Could you check a few things on this model? Use its own coordinates, in mm. A direction names the side the tool comes from. Give positions to 0.01 mm unless a question says otherwise; leave off trailing zeros. Loops run counter-clockwise (first coordinate to the right, second up) from the corner with the lowest first, then second, coordinate; pieces in that order, holes last. Notation, with made-up numbers: (-4.5, 66.25) - (19.5, 66.25) arc R29 ccw to (19.5, 104.25) - close; hole circle Ø3 at (-24, 39). An arc over 180 degrees is marked (long way). Answer in a Markdown table with one row per item. Add a question column.
```python
from build123d import *

# Parameters (mm, degrees)
F0_W          = 152
F0_H          = 55
F1_DEPTH      = 39
F2_W          = 53
F2_H          = 34
F3_DEPTH      = 150
F5_DEPTH      = 10.9
F7_DEPTH      = 100
F8_DEPTH      = 5
F9_DEPTH      = 4
F10_DEPTH     = 5
F11_DEPTH     = 5
F12_DEPTH     = 5
F13_W         = 8
F13_H         = 4
F14_DEPTH     = 100
F15_T1_DEPTH  = 163.5
F15_T3_DEPTH  = 74
F15_T5_DEPTH  = 56.5
F15_T7_DEPTH  = 55
F15_S11_W     = 5
F15_S11_H     = 5
F15_T12_DEPTH = 5
F15_S17_W     = 5
F15_S17_H     = 5
F15_T18_DEPTH = 5
F16_W         = 7.2434431314
F16_H         = 13.5
F16_W_2       = 55
F16_W_3       = 10.0454574823
F17_DEPTH     = 6
F18_R         = 5
F19_W         = 10
F19_H         = 4
F20_DEPTH     = 38.8


# Not quite as in the source:
# - a fillet or chamfer that OpenCascade refuses, or shapes differently, is made with other operations: its cross-section is extruded or revolved along the edge and cut away or added


with BuildPart() as f1:
    # F0 (on Top) → F1 (new body)
    with BuildSketch(Plane.XY):
        Rectangle(F0_W, F0_H)
    extrude(amount=F1_DEPTH)

    # F2 (on face) → F3 (cut)
    with BuildSketch(Plane(origin=(-76, 0, 0), x_dir=(0, -1, 0), z_dir=(-1, 0, 0))):
        with Locations((0, 19.5)):
            Rectangle(F2_W, F2_H)
    extrude(amount=-F3_DEPTH, mode=Mode.SUBTRACT)

    # F4 (on face) → F5 (cut)
    with BuildSketch(Plane(origin=(0, 0, 0), x_dir=(1, 0, 0), z_dir=(0, 0, -1))):
        with BuildLine():
            ThreePointArc((-29.5, 16.5), (-30.9644660941, 20.0355339059), (-34.5, 21.5))
            Line((-34.5, 21.5), (-59.5, 21.5))
            ThreePointArc((-59.5, 21.5), (-63.0355339059, 20.0355339059), (-64.5, 16.5))
            Line((-64.5, 16.5), (-64.5, -16.5))
            ThreePointArc((-64.5, -16.5), (-63.0355339059, -20.0355339059), (-59.5, -21.5))
            Line((-59.5, -21.5), (-34.5, -21.5))
            ThreePointArc((-34.5, -21.5), (-30.9644660941, -20.0355339059), (-29.5, -16.5))
            Line((-29.5, -16.5), (-29.5, 16.5))
        make_face()
        with BuildLine():
            Line((-12.5, -21.5), (12.5, -21.5))
            ThreePointArc((12.5, -21.5), (16.0355339059, -20.0355339059), (17.5, -16.5))
            Line((17.5, -16.5), (17.5, 16.5))
            ThreePointArc((17.5, 16.5), (16.0355339059, 20.0355339059), (12.5, 21.5))
            Line((12.5, 21.5), (-12.5, 21.5))
            ThreePointArc((-12.5, 21.5), (-16.0355339059, 20.0355339059), (-17.5, 16.5))
            Line((-17.5, 16.5), (-17.5, -16.5))
            ThreePointArc((-17.5, -16.5), (-16.0355339059, -20.0355339059), (-12.5, -21.5))
        make_face()
        with BuildLine():
            ThreePointArc((64.5, 16.5), (63.0355339059, 20.0355339059), (59.5, 21.5))
            Line((59.5, 21.5), (34.5, 21.5))
            ThreePointArc((34.5, 21.5), (30.9644660941, 20.0355339059), (29.5, 16.5))
            Line((29.5, 16.5), (29.5, -16.5))
            ThreePointArc((29.5, -16.5), (30.9644660941, -20.0355339059), (34.5, -21.5))
            Line((34.5, -21.5), (59.5, -21.5))
            ThreePointArc((59.5, -21.5), (63.0355339059, -20.0355339059), (64.5, -16.5))
            Line((64.5, -16.5), (64.5, 16.5))
        make_face()
    extrude(amount=-F5_DEPTH, mode=Mode.SUBTRACT)

    # F6 (on face) → F7 (cut)
    with BuildSketch(Plane.XZ.offset(27.5)):
        with BuildLine():
            ThreePointArc((-28, 29.5), (-29.4644660941, 33.0355339059), (-33, 34.5))
            Line((-33, 34.5), (-63, 34.5))
            ThreePointArc((-63, 34.5), (-66.5355339059, 33.0355339059), (-68, 29.5))
            Line((-68, 29.5), (-68, 9.5))
            ThreePointArc((-68, 9.5), (-66.5355339059, 5.9644660941), (-63, 4.5))
            Line((-63, 4.5), (-33, 4.5))
            ThreePointArc((-33, 4.5), (-29.4644660941, 5.9644660941), (-28, 9.5))
            Line((-28, 9.5), (-28, 29.5))
        make_face()
        with BuildLine():
            ThreePointArc((20, 29.5), (18.5355339059, 33.0355339059), (15, 34.5))
            Line((15, 34.5), (-15, 34.5))
            ThreePointArc((-15, 34.5), (-18.5355339059, 33.0355339059), (-20, 29.5))
            Line((-20, 29.5), (-20, 9.5))
            ThreePointArc((-20, 9.5), (-18.5355339059, 5.9644660941), (-15, 4.5))
            Line((-15, 4.5), (15, 4.5))
            ThreePointArc((15, 4.5), (18.5355339059, 5.9644660941), (20, 9.5))
            Line((20, 9.5), (20, 29.5))
        make_face()
        with BuildLine():
            ThreePointArc((58, 29.5), (56.5355339059, 33.0355339059), (53, 34.5))
            Line((53, 34.5), (33, 34.5))
            ThreePointArc((33, 34.5), (29.4644660941, 33.0355339059), (28, 29.5))
            Line((28, 29.5), (28, 9.5))
            ThreePointArc((28, 9.5), (29.4644660941, 5.9644660941), (33, 4.5))
            Line((33, 4.5), (53, 4.5))
            ThreePointArc((53, 4.5), (56.5355339059, 5.9644660941), (58, 9.5))
            Line((58, 9.5), (58, 29.5))
        make_face()
    extrude(amount=-F7_DEPTH, mode=Mode.SUBTRACT)

    # F8 (add): a face of the model
    f8_faces = [f1.faces().sort_by_distance(p)[0] for p in [
        (0, 0, 39),
    ]]
    extrude(f8_faces, amount=F8_DEPTH)

    # F9 (add): a face of the model
    f9_faces = [f1.faces().sort_by_distance(p)[0] for p in [
        (76, 0, 22),
    ]]
    extrude(f9_faces, amount=F9_DEPTH)

    # F10 (add): a face of the model
    f10_faces = [f1.faces().sort_by_distance(p)[0] for p in [
        (2, 0, 44),
    ]]
    extrude(f10_faces, amount=F10_DEPTH)

    # F11 (add): a face of the model
    f11_faces = [f1.faces().sort_by_distance(p)[0] for p in [
        (-74.3648547465, 27.5, 24.5),
    ]]
    extrude(f11_faces, amount=F11_DEPTH)

    # F12 (add): a face of the model
    f12_faces = [f1.faces().sort_by_distance(p)[0] for p in [
        (-74.3648547465, -27.5, 24.5),
    ]]
    extrude(f12_faces, amount=F12_DEPTH)

    # F13 (on face) → F14 (cut)
    with BuildSketch(Plane.XZ.offset(32.5)):
        with Locations((-26, 43.8039299548)):
            Rectangle(F13_W, F13_H)
        with Locations((10, 43.8039299548)):
            Rectangle(F13_W, F13_H)
        with Locations((63, 43.8039299548)):
            Rectangle(F13_W, F13_H)
    extrude(amount=-F14_DEPTH, mode=Mode.SUBTRACT)

    # F15: fillet of radius 5 on 7 edges, made by hand

    # F15_s2 → F15_t1 (cut)
    with BuildSketch(Plane.YZ.offset(-71)):
        with BuildLine():
            ThreePointArc((-27.5, 0), (-31.0355339059, 1.4644660941), (-32.5, 5))
            Line((-32.5, 5), (-32.5, 0))
            Line((-32.5, 0), (-27.5, 0))
        make_face()
        with BuildLine():
            ThreePointArc((27.5, 0), (31.0355339059, 1.4644660941), (32.5, 5))
            Line((32.5, 5), (32.5, 0))
            Line((32.5, 0), (27.5, 0))
        make_face()
    extrude(amount=F15_T1_DEPTH, mode=Mode.SUBTRACT)

    # F15_s4 → F15_t3 (cut)
    with BuildSketch(Plane.XY.offset(-12.5)):
        with BuildLine():
            ThreePointArc((80, 27.5), (78.5355339059, 31.0355339059), (75, 32.5))
            Line((75, 32.5), (80, 32.5))
            Line((80, 32.5), (80, 27.5))
        make_face()
        with BuildLine():
            ThreePointArc((80, -27.5), (78.5355339059, -31.0355339059), (75, -32.5))
            Line((75, -32.5), (80, -32.5))
            Line((80, -32.5), (80, -27.5))
        make_face()
    extrude(amount=F15_T3_DEPTH, mode=Mode.SUBTRACT)

    # F15_s6 → F15_t5 (cut)
    with BuildSketch(Plane.XY.offset(5)):
        with BuildLine():
            ThreePointArc((-76, -27.5), (-74.5355339059, -31.0355339059), (-71, -32.5))
            Line((-71, -32.5), (-76, -32.5))
            Line((-76, -32.5), (-76, -27.5))
        make_face()
        with BuildLine():
            ThreePointArc((-71, 32.5), (-74.5355339059, 31.0355339059), (-76, 27.5))
            Line((-76, 27.5), (-76, 32.5))
            Line((-76, 32.5), (-71, 32.5))
        make_face()
    extrude(amount=F15_T5_DEPTH, mode=Mode.SUBTRACT)

    # F15_s8 → F15_t7 (cut)
    with BuildSketch(Plane.XZ.offset(-27.5)):
        with BuildLine():
            ThreePointArc((-71, 0), (-74.5355339059, 1.4644660941), (-76, 5))
            Line((-76, 5), (-76, 0))
            Line((-76, 0), (-71, 0))
        make_face()
    extrude(amount=F15_T7_DEPTH, mode=Mode.SUBTRACT)


with BuildPart() as f15_tool10:
    # F15_s11 → F15_t12 (new body)
    with BuildSketch(Plane.XY.offset(5)):
        with Locations((-73.5, -30)):
            Rectangle(F15_S11_W, F15_S11_H)
    extrude(amount=-F15_T12_DEPTH)

    # F15_s13 → F15_t14 (revolve, cut)
    with BuildSketch(Plane(origin=(-71, -27.5, 5), x_dir=(0.7071067812, 0.7071067812, 0), z_dir=(-0.7071067812, 0.7071067812, 0))):
        with BuildLine():
            ThreePointArc((0, -5), (5, 0), (0, 5))
            Line((0, 5), (0, -5))
        make_face()
    revolve(axis=Axis((-71, -27.5, 5), (0, 0, -1)), mode=Mode.SUBTRACT)


with BuildPart() as f1_1:
    add(f1.part)

    # F15_t9: cut F15_tool10
    add(f15_tool10.part, mode=Mode.SUBTRACT)


with BuildPart() as f15_tool16:
    # F15_s17 → F15_t18 (new body)
    with BuildSketch(Plane.XY.offset(5)):
        with Locations((-73.5, 30)):
            Rectangle(F15_S17_W, F15_S17_H)
    extrude(amount=-F15_T18_DEPTH)

    # F15_s19 → F15_t20 (revolve, cut)
    with BuildSketch(Plane(origin=(-71, 27.5, 5), x_dir=(0.7071067812, -0.7071067812, 0), z_dir=(0.7071067812, 0.7071067812, 0))):
        with BuildLine():
            ThreePointArc((0, -5), (5, 0), (0, 5))
            Line((0, 5), (0, -5))
        make_face()
    revolve(axis=Axis((-71, 27.5, 5), (0, 0, -1)), mode=Mode.SUBTRACT)


with BuildPart() as f1_2:
    add(f1_1.part)

    # F15_t15: cut F15_tool16
    add(f15_tool16.part, mode=Mode.SUBTRACT)

    # F16 (on face) → F17 (cut)
    with BuildSketch(Plane.YZ.offset(80)):
        with Locations((-31.1217215657, 21.25)):
            Rectangle(F16_W, F16_H)
        with Locations((0, 21.25)):
            Rectangle(F16_W_2, F16_H)
        with Locations((32.5227287412, 21.25)):
            Rectangle(F16_W_3, F16_H)
    extrude(amount=-F17_DEPTH, mode=Mode.SUBTRACT)

    # F18
    f18_edges = [f1_2.edges().sort_by_distance(p)[0] for p in [
        (74, -32.5, 21.25),
        (74, 32.5, 21.25),
        (80, 0, 28),
        (80, 0, 14.5),
    ]]
    fillet(f18_edges, radius=F18_R)

    # F19 (on face) → F20 (cut)
    with BuildSketch(Plane(origin=(-76, 0, 0), x_dir=(0, -1, 0), z_dir=(-1, 0, 0))):
        with Locations((9.5, 47)):
            Rectangle(F19_W, F19_H)
    extrude(amount=-F20_DEPTH, mode=Mode.SUBTRACT)


solid = f1_2.part
```
(1) I want a section at D-D on z = 6.5. State how many separate pieces and enclosed holes the cut face has, then the cut area to 3 significant figures.
(2) Please list where these lines run through material, in increasing order: line 1 (X direction, y = 23, z = 43.5); line 2 (Y direction, x = 67, z = 22.5); line 3 (Z direction, x = -43.5, y = 22.5).
(3) I want a section at C-C on x = 8. Please give me the cut outline in (y, z).
(4) For pin 1 Ø6.5 at (x, y) = (-26.5, 7) entering from -Z; pin 2 Ø6 at (x, y) = (60, -14.5) entering from -Z; pin 3 Ø1.2 at (y, z) = (-10, 47) entering from -X; pin 4 Ø2 at (y, z) = (4, 1) entering from -X, each with a flat end and sliding along its axis, tell me the tip position at first contact or that it passes through.
(5) I want a section at A-A on y = -23.5. Please give me the cut outline in (x, z).
(6) On a 3-axis mill with a long thin cutter (end or side, diameter ignored), from which of +Z, -Z, +X, -X, +Y, -Y can I reach the whole of each face in a straight line? I mean faces 1 (the cylindrical face through (73.291, 31.564, 12.413)), 2 (the flat face through (74, 0, 32)), 3 (the cylindrical face through (78.57, 31, 40.89)), 4 (the cylindrical face through (-16.07, 20, 1.23)), 5 (the flat face through (0, -29, 4.5)). Say none if no direction works.
(7) We'd pull the mould along Z, two halves only. Please class faces 6 (the flat face through (58, -29, 19)), 7 (the cylindrical face through (30.93, 20, 1.23)): pulls with the +Z half, pulls with the -Z half, needs draft (parallel to the pull), parting line crosses it, or undercut.
(8) I want a section at B-B on x = -44. Please give me the cut outline in (y, z), then the cut area to 3 significant figures.
Reported:
| question | item | result |
|---|---|---|
| 1 | separate pieces | 7 |
| 1 | enclosed holes | 0 |
| 1 | area | 921 mm² |
| 2 | line 1 | -76 to -30, -22 to 6, 14 to 59, 67 to 80 |
| 2 | line 2 | -32.5 to -26.5, 26.5 to 32.5 |
| 2 | line 3 | 0 to 2.5, 36.5 to 49 |
| 3 | outline | (-32.5, 34.5) - (-26.5, 34.5) - (-26.5, 36.5) - (26.5, 36.5) - (26.5, 34.5) - (32.5, 34.5) - (32.5, 41.8) - (-32.5, 41.8) - close; (-32.5, 45.8) - (32.5, 45.8) - (32.5, 49) - (-32.5, 49) - close; (-32.47, 4.5) arc R5 ccw to (-27.5, 0) - (-21.5, 0) - (-21.5, 2.5) - (-26.5, 2.5) - (-26.5, 4.5) - close; (21.5, 0) - (27.5, 0) arc R5 ccw to (32.47, 4.5) - (26.5, 4.5) - (26.5, 2.5) - (21.5, 2.5) - close |
| 4 | pin 1 | z = 0 |
| 4 | pin 2 | z = 36.5 |
| 4 | pin 3 | x = -37.2 |
| 4 | pin 4 | x = -75 |
| 5 | outline | (-76, 36.5) - (74, 36.5) - (74, 28) - (75, 28) arc R5 ccw to (80, 33) - (80, 49) - (-76, 49) - close; (-75.33, 2.5) arc R5 ccw to (-71, 0) - (80, 0) - (80, 9.5) arc R5 ccw to (75, 14.5) - (74, 14.5) - (74, 2.5) - close; hole (-30, 41.8) - (-22, 41.8) - (-22, 45.8) - (-30, 45.8) - close; hole (6, 41.8) - (14, 41.8) - (14, 45.8) - (6, 45.8) - close; hole (59, 41.8) - (67, 41.8) - (67, 45.8) - (59, 45.8) - close |
| 6 | face 1 | +X, +Y |
| 6 | face 2 | -X |
| 6 | face 3 | +Z, -Z, +X, +Y |
| 6 | face 4 | -Z |
| 6 | face 5 | +Y, -Y |
| 7 | face 6 | undercut |
| 7 | face 7 | needs draft |
| 8 | outline | (-32.5, 34.5) - (-26.5, 34.5) - (-26.5, 36.5) - (26.5, 36.5) - (26.5, 34.5) - (32.5, 34.5) - (32.5, 49) - (-4.5, 49) - (-4.5, 45) - (-14.5, 45) - (-14.5, 49) - (-32.5, 49) - close; (-32.47, 4.5) arc R5 ccw to (-27.5, 0) - (-21.5, 0) - (-21.5, 2.5) - (-26.5, 2.5) - (-26.5, 4.5) - close; (21.5, 0) - (27.5, 0) arc R5 ccw to (32.47, 4.5) - (26.5, 4.5) - (26.5, 2.5) - (21.5, 2.5) - close |
| 8 | area | 865 mm² |
